```python
from build123d import *

# Parameters (mm, degrees)
SKETCH1_W                                           = 420
SKETCH1_H                                           = 190
BOSS_EXTRUDE1_DEPTH                                 = 12.7
FILLET1_R                                           = 10
SKETCH8_R                                           = 44.45
CUT_EXTRUDE1_DEPTH                                  = 4
SKETCH8_3_R                                         = 25.5
CUT_EXTRUDE2_DEPTH                                  = 13.7
CBORE_FOR_8_BINDING_HEAD_MACHINE_SCREW1_D           = 4.499991
CBORE_FOR_8_BINDING_HEAD_MACHINE_SCREW1_DEPTH       = 10
CBORE_FOR_8_BINDING_HEAD_MACHINE_SCREW1_CBORE_D     = 8.2499962
CBORE_FOR_8_BINDING_HEAD_MACHINE_SCREW1_CBORE_DEPTH = 3.999992
CBORE_FOR_8_BINDING_HEAD_MACHINE_SCREW1_TIP         = 1.351933689
CUT_EXTRUDE3_DEPTH                                  = 13.7
TAP_DRILL_FOR_M4X0_7_TAP1_D                         = 3.3
SKETCH18_W                                          = 135
SKETCH18_H                                          = 190
CUT_EXTRUDE4_DEPTH                                  = 13.7
FILLET2_R                                           = 10
SKETCH25_W                                          = 38.190452802
SKETCH25_H                                          = 150
CUT_EXTRUDE5_DEPTH                                  = 13.7
SKETCH26_W                                          = 40
SKETCH26_H                                          = 150
CUT_EXTRUDE6_DEPTH                                  = 13.7
FILLET4_R                                           = 10
CUT_EXTRUDE8_DEPTH                                  = 1
CUT_EXTRUDE8_DEPTH_BACK                             = 13.7
FILLET6_R                                           = 10
M5_CLEARANCE_HOLE4_D                                = 5.5
BOSS_EXTRUDE4_DEPTH                                 = 12.7
SKETCH42_W                                          = 246.809547198
SKETCH42_H                                          = 6.096
CUT_EXTRUDE9_DEPTH                                  = 12.7
FILLET7_R                                           = 10


with BuildPart() as part:
    # Sketch1 → Boss-Extrude1 (new body)
    with BuildSketch(Plane.XY):
        Rectangle(SKETCH1_W, SKETCH1_H)
    extrude(amount=BOSS_EXTRUDE1_DEPTH)

    # Fillet1
    fillet1_edges = [part.edges().sort_by_distance(p)[0] for p in [
        (210, -95, 6.35),
        (-210, -95, 6.35),
        (-210, 95, 6.35),
        (210, 95, 6.35),
    ]]
    fillet(fillet1_edges, radius=FILLET1_R)

    # Sketch8 → Cut-Extrude1 (cut)
    with BuildSketch(Plane.XY.offset(12.7)):
        Circle(SKETCH8_R)
    extrude(amount=-CUT_EXTRUDE1_DEPTH, mode=Mode.SUBTRACT)

    # Sketch8<3> → Cut-Extrude2 (cut, through all)
    with BuildSketch(Plane.XY.offset(12.7)):
        Circle(SKETCH8_3_R)
    extrude(amount=-CUT_EXTRUDE2_DEPTH, mode=Mode.SUBTRACT)

    # CBORE for #8 Binding Head Machine Screw1
    with Locations(Plane(origin=(0, 0, 0), x_dir=(-1, 0, 0), z_dir=(0, 0, -1))):
        with Locations((0, 41), (0, -41), (28.991378029, -28.991378029), (-28.991378029, -28.991378029), (-41, 0), (41, 0), (-28.991378029, 28.991378029), (28.991378029, 28.991378029)):
            CounterBoreHole(CBORE_FOR_8_BINDING_HEAD_MACHINE_SCREW1_D / 2, CBORE_FOR_8_BINDING_HEAD_MACHINE_SCREW1_CBORE_D / 2, CBORE_FOR_8_BINDING_HEAD_MACHINE_SCREW1_CBORE_DEPTH, depth=CBORE_FOR_8_BINDING_HEAD_MACHINE_SCREW1_DEPTH)
            with Locations((0, 0, -(CBORE_FOR_8_BINDING_HEAD_MACHINE_SCREW1_DEPTH + CBORE_FOR_8_BINDING_HEAD_MACHINE_SCREW1_TIP / 2))):  # 118° drill point
                Cone(0, CBORE_FOR_8_BINDING_HEAD_MACHINE_SCREW1_D / 2, CBORE_FOR_8_BINDING_HEAD_MACHINE_SCREW1_TIP, mode=Mode.SUBTRACT)

    # Sketch12 → Cut-Extrude3 (cut, through all)
    with BuildSketch(Plane.XY.offset(12.7)):
        with BuildLine():
            Line((119, -18.5), (129, -18.5))
            ThreePointArc((129, -18.5), (147.5, 0), (129, 18.5))
            Line((129, 18.5), (119, 18.5))
            ThreePointArc((119, 18.5), (100.5, 0), (119, -18.5))
        make_face()
    extrude(amount=-CUT_EXTRUDE3_DEPTH, mode=Mode.SUBTRACT)

    # Tap Drill for M4x0.7 Tap1 (through all)
    with Locations(Plane.XY.offset(12.7)):
        with Locations((111.75, 25.5), (136.25, 25.5), (111.75, -25.5), (136.25, -25.5)):
            Hole(TAP_DRILL_FOR_M4X0_7_TAP1_D / 2)

    # Sketch18 → Cut-Extrude4 (cut, through all)
    with BuildSketch(Plane.XY.offset(12.7)):
        with Locations((-142.5, 0)):
            Rectangle(SKETCH18_W, SKETCH18_H)
    extrude(amount=-CUT_EXTRUDE4_DEPTH, mode=Mode.SUBTRACT)

    # Fillet2
    fillet2_edges = [part.edges().sort_by_distance(p)[0] for p in [
        (-75, 95, 6.35),
        (-75, -95, 6.35),
    ]]
    fillet(fillet2_edges, radius=FILLET2_R)

    # Sketch25 → Cut-Extrude5 (cut, through all)
    with BuildSketch(Plane.XY.offset(12.7)):
        with Locations((190.904773599, 0)):
            Rectangle(SKETCH25_W, SKETCH25_H)
    extrude(amount=-CUT_EXTRUDE5_DEPTH, mode=Mode.SUBTRACT)

    # Sketch26 → Cut-Extrude6 (cut, through all)
    with BuildSketch(Plane.XY.offset(12.7)):
        with Locations((70.340308105, 0)):
            Rectangle(SKETCH26_W, SKETCH26_H)
    extrude(amount=-CUT_EXTRUDE6_DEPTH, mode=Mode.SUBTRACT)

    # Fillet4
    fillet4_edges = [part.edges().sort_by_distance(p)[0] for p in [
        (90.340308105, 75, 6.35),
        (90.340308105, -75, 6.35),
        (50.340308105, -75, 6.35),
        (50.340308105, 75, 6.35),
    ]]
    fillet(fillet4_edges, radius=FILLET4_R)

    # Sketch35 → Cut-Extrude8 (cut, two sides)
    with BuildSketch(Plane.XY.offset(12.7)) as cut_extrude8_sk:
        Polygon((171.809547198, -75), (171.809547198, -95), (219.38654528, -95), (219.38654528, 95), (171.809547198, 95), align=None)
    extrude(amount=CUT_EXTRUDE8_DEPTH, mode=Mode.SUBTRACT)
    extrude(cut_extrude8_sk.sketch, amount=-CUT_EXTRUDE8_DEPTH_BACK, mode=Mode.SUBTRACT)

    # Fillet6
    fillet6_edges = [part.edges().sort_by_distance(p)[0] for p in [
        (171.809547198, -95, 6.35),
        (171.809547198, 95, 6.35),
    ]]
    fillet(fillet6_edges, radius=FILLET6_R)

    # M5 Clearance Hole4 (through all)
    with Locations(Plane.XY.offset(12.7)):
        with Locations((161.809547198, -71.25), (161.809547198, -47.5), (161.809547198, -23.75), (161.809547198, 0), (161.809547198, 23.75), (161.809547198, 47.5), (161.809547198, 71.25), (-65, 71.25), (-65, 47.5), (-65, 23.75), (-65, 0), (-65, -23.75), (-65, -47.5), (-65, -71.25)):
            Hole(M5_CLEARANCE_HOLE4_D / 2)

    # Sketch41 → Boss-Extrude4 (add)
    with BuildSketch(Plane(origin=(0, 0, 0), x_dir=(-1, 0, 0), z_dir=(0, 0, -1))):
        with BuildLine():
            Line((75, 85), (75, 95))
            Line((75, 95), (65, 95))
            ThreePointArc((65, 95), (72.071067812, 92.071067812), (75, 85))
        make_face()
        with BuildLine():
            Line((75, -95), (65, -95))
            ThreePointArc((65, -95), (72.071067812, -92.071067812), (75, -85))
            Line((75, -85), (75, -95))
        make_face()
        with BuildLine():
            Line((-171.809547198, -85), (-171.809547198, -95))
            Line((-171.809547198, -95), (-161.809547198, -95))
            ThreePointArc((-161.809547198, -95), (-168.88061501, -92.071067812), (-171.809547198, -85))
        make_face()
        with BuildLine():
            Line((-171.809547198, 95), (-161.809547198, 95))
            ThreePointArc((-161.809547198, 95), (-168.88061501, 92.071067812), (-171.809547198, 85))
            Line((-171.809547198, 85), (-171.809547198, 95))
        make_face()
    extrude(amount=-BOSS_EXTRUDE4_DEPTH)

    # Sketch42 → Cut-Extrude9 (cut)
    with BuildSketch(Plane(origin=(0, 0, 0), x_dir=(-1, 0, 0), z_dir=(0, 0, -1))):
        with Locations((-48.404773599, 91.952)):
            Rectangle(SKETCH42_W, SKETCH42_H)
        with Locations((-48.404773599, -91.952)):
            Rectangle(SKETCH42_W, SKETCH42_H)
    extrude(amount=-CUT_EXTRUDE9_DEPTH, mode=Mode.SUBTRACT)

    # Fillet7
    fillet7_edges = [part.edges().sort_by_distance(p)[0] for p in [
        (171.809547198, 88.904, 6.35),
        (-75, 88.904, 6.35),
        (-75, -88.904, 6.35),
        (171.809547198, -88.904, 6.35),
    ]]
    fillet(fillet7_edges, radius=FILLET7_R)


solid = part.part
```
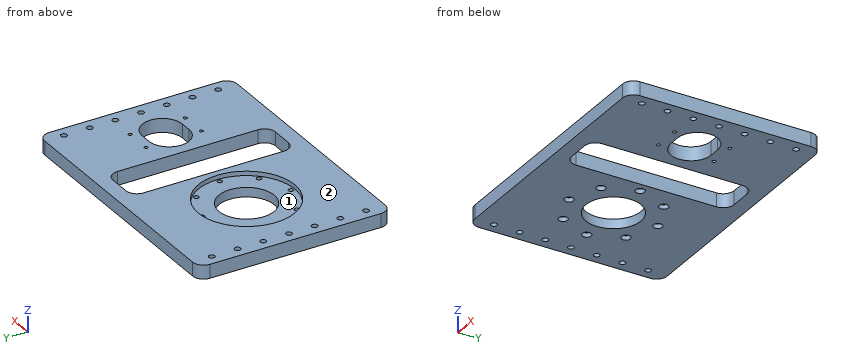
Geometry check sheet. Reference: the model listing, model coordinates, mm. Face numbers are marked on the shaded views. Round coordinates to 2 decimals unless told otherwise and drop trailing zeros. Write each loop counter-clockwise with the first axis right and the second up, starting at its lowest first coordinate (ties: lowest second). Pieces come first, ordered by that corner, then holes. Notation, with made-up numbers: (-39, 54.25) - (-11, 54.25) arc R25 cw to (-11, 84.25) - close; hole circle Ø7 at (-5, -2.5). An arc over 180 degrees is marked (long way). Write each question's results on one line, items separated by ' | '.
(1) Thickness scan on probe 1 along Y at (x, z) = (119.5, 7.5); probe 2 along X at (y, z) = (-61, 0.75); probe 3 along X at (y, z) = (-3, 4.25). Record the ranges inside material, lowest first. Write a range as from..to.
Computed:
probe 1: y = -88.9..-18.5, 18.5..88.9 | probe 2: x = -75..50.34, 90.34..171.81 | probe 3: x = -75..-25.32, 25.32..50.34, 90.34..100.74, 147.26..171.81
(2) Sectioned sample at A-A, the plane x = 69.5. Enter the section's corners in (y, z).
Computed:
outline: (-88.9, 0) - (-75, 0) - (-75, 12.7) - (-88.9, 12.7) - close; (75, 0) - (88.9, 0) - (88.9, 12.7) - (75, 12.7) - close
(3) Depth check by flat-ended pin: pin 1 Ø4 at (x, y) = (0, 41) entering from -Z; pin 2 Ø6 at (x, y) = (41, 0) entering from +Z; pin 3 Ø4 at (x, y) = (-0.5, 40.5) entering from -Z. Enter the tip coordinate at first touch or a pass-through.
Computed:
pin 1: passes through | pin 2: stops at z = 8.7 | pin 3: stops at z = 4
(4) Sectioned sample at B-B, the plane y = -71.25. Enter the section's corners in (x, z).
Computed:
outline: (-75, 0) - (-67.75, 0) - (-67.75, 12.7) - (-75, 12.7) - close; (-62.25, 0) - (52.53, 0) - (52.53, 12.7) - (-62.25, 12.7) - close; (88.15, 0) - (159.06, 0) - (159.06, 12.7) - (88.15, 12.7) - close; (164.56, 0) - (171.81, 0) - (171.81, 12.7) - (164.56, 12.7) - close
(5) Draft check along Y on the marked faces 1 and 2. Enter one of: pulls with the +Y half, pulls with the -Y half, needs draft (parallel to the pull), parting line crosses it, or undercut.
Computed:
face 1: undercut | face 2: needs draft
